Check sheet for the modelled part. Datum: model origin and axes. Units: mm. A direction names the side the tool comes from. Coordinates: 2 decimals unless noted, no trailing zeros. Loops run counter-clockwise (first coordinate to the right, second up) from the corner with the lowest first, then second, coordinate; pieces in that order, holes last.
```python
from build123d import *

# Parameters (mm, degrees)
CROQUIS1_R                               = 7.5
CROQUIS1_R_2                             = 4
SALIENTE_EXTRUIR1_DEPTH                  = 15
CROQUIS2_W                               = 3
CROQUIS2_H                               = 16.302446726
CORTAR_EXTRUIR1_DEPTH                    = 3
SALIENTE_EXTRUIR2_START                  = 5
SALIENTE_EXTRUIR2_DEPTH                  = 5
TALADRO_DE_MARGEN_PARA_M1_61_D           = 1.7
TALADRO_DE_MARGEN_PARA_M1_61_CSINK_D     = 1.75
TALADRO_DE_MARGEN_PARA_M1_61_CSINK_ANGLE = 82
REDONDEO1_R                              = 2
SALIENTE_EXTRUIR3_DEPTH                  = 5


# Read off the part's stored shape, not the designer's step: M14x1.5 Roscas Standard Taladro1
with BuildPart() as part:
    # Croquis1 → Saliente-Extruir1 (new body)
    with BuildSketch(Plane(origin=(0, 0, 0), x_dir=(1, 0, 0), z_dir=(0, 1, 0))):
        with Locations(Location((0, 0, 0), (0, 0, 270))):
            Circle(CROQUIS1_R)
        with Locations(Location((0, 0, 0), (0, 0, 270))):
            Circle(CROQUIS1_R_2, mode=Mode.SUBTRACT)
    extrude(amount=SALIENTE_EXTRUIR1_DEPTH)

    # Croquis2 → Cortar-Extruir1 (cut)
    with BuildSketch(Plane(origin=(0, 15, 0), x_dir=(1, 0, 0), z_dir=(0, 1, 0))):
        Rectangle(CROQUIS2_W, CROQUIS2_H)
    extrude(amount=-CORTAR_EXTRUIR1_DEPTH, mode=Mode.SUBTRACT)

    # M14x1.5 Roscas Standard Taladro1 outline → M14x1.5 Roscas Standard Taladro1 (revolve, cut)
    with BuildSketch(Plane.XY):
        Polygon((6.172, 0), (7.5, 0), (7.5, 10), (7, 10), (7, 0.828), align=None)
    revolve(axis=Axis((0, 0, 0), (0, 1, 0)), mode=Mode.SUBTRACT)

    # Croquis4 → Saliente-Extruir2 (add)
    with BuildSketch(Plane.XZ.offset(SALIENTE_EXTRUIR2_START)):
        with BuildLine():
            ThreePointArc((2.645751311, -3), (3.409321836, -2.092014488), (3.872983346, -1))
            Line((3.872983346, -1), (-3.872983346, -1))
            ThreePointArc((-3.872983346, -1), (-3.409321836, -2.092014488), (-2.645751311, -3))
            Line((-2.645751311, -3), (2.645751311, -3))
        make_face()
        with BuildLine():
            Line((-3.872983346, 1), (3.872983346, 1))
            ThreePointArc((3.872983346, 1), (3.409321836, 2.092014488), (2.645751311, 3))
            Line((2.645751311, 3), (-2.645751311, 3))
            ThreePointArc((-2.645751311, 3), (-3.409321836, 2.092014488), (-3.872983346, 1))
        make_face()
        with BuildLine():
            Line((3.872983346, 1), (5.074404793, 1))
            ThreePointArc((5.074404793, 1), (4.750167411, 2.045847884), (4.213025516, 3))
            Line((4.213025516, 3), (2.645751311, 3))
            ThreePointArc((2.645751311, 3), (3.409321836, 2.092014488), (3.872983346, 1))
        make_face()
        with BuildLine():
            Line((-5.074404793, 1), (-3.872983346, 1))
            ThreePointArc((-3.872983346, 1), (-3.409321836, 2.092014488), (-2.645751311, 3))
            Line((-2.645751311, 3), (-4.213025516, 3))
            ThreePointArc((-4.213025516, 3), (-4.750167411, 2.045847884), (-5.074404793, 1))
        make_face()
        with BuildLine():
            ThreePointArc((4.213025516, -3), (4.750167411, -2.045847884), (5.074404793, -1))
            Line((5.074404793, -1), (3.872983346, -1))
            ThreePointArc((3.872983346, -1), (3.409321836, -2.092014488), (2.645751311, -3))
            Line((2.645751311, -3), (4.213025516, -3))
        make_face()
        with BuildLine():
            ThreePointArc((-2.645751311, -3), (-3.409321836, -2.092014488), (-3.872983346, -1))
            Line((-3.872983346, -1), (-5.074404793, -1))
            ThreePointArc((-5.074404793, -1), (-4.750167411, -2.045847884), (-4.213025516, -3))
            Line((-4.213025516, -3), (-2.645751311, -3))
        make_face()
    extrude(amount=-SALIENTE_EXTRUIR2_DEPTH)

    # Taladro de margen para M1.61 (through all)
    with Locations(Plane(origin=(0, 0, -3), x_dir=(1, 0, 0), z_dir=(0, 0, -1))):
        with Locations((2.65, 2.5), (-2.65, 2.5)):
            CounterSinkHole(TALADRO_DE_MARGEN_PARA_M1_61_D / 2, TALADRO_DE_MARGEN_PARA_M1_61_CSINK_D / 2, counter_sink_angle=TALADRO_DE_MARGEN_PARA_M1_61_CSINK_ANGLE)

    # Redondeo1
    # the kernel refuses this fillet: 2 mm, written as the material it adds along each edge
    with BuildSketch(Plane(origin=(0, 0, 0), x_dir=(0.503234651569935, 0, -0.8641498049871251), z_dir=(0.8641498049871251, 0, 0.503234651569935))) as redondeo1_piece_1_section:
        with BuildLine():
            CenterArc((4 - REDONDEO1_R, REDONDEO1_R), REDONDEO1_R, 270, 90)
            Line((4 - REDONDEO1_R, 0), (4, 0))
            Line((4, 0), (4, REDONDEO1_R))
        make_face()
    redondeo1_piece_1 = revolve(axis=Axis((0, 0, 0), (0, 1, 0)), revolution_arc=177.360579055, mode=Mode.PRIVATE)
    redondeo1_piece_1 = split(redondeo1_piece_1, bisect_by=Plane(origin=(0.549602468, 0.055077536, -1), z_dir=(0, 0, -1)), keep=Keep.TOP, mode=Mode.PRIVATE)
    redondeo1_piece_1 = split(redondeo1_piece_1, bisect_by=Plane(origin=(0.549602468, 0.055077536, -3), z_dir=(0, 0, 1)), keep=Keep.TOP, mode=Mode.PRIVATE)
    add(redondeo1_piece_1)
    with BuildSketch(Plane(origin=(0, 0, 0), x_dir=(0.503234651569935, 0, -0.8641498049871251), z_dir=(0.8641498049871251, 0, 0.503234651569935))) as redondeo1_piece_2_section:
        with BuildLine():
            CenterArc((4 - REDONDEO1_R, REDONDEO1_R), REDONDEO1_R, 270, 90)
            Line((4 - REDONDEO1_R, 0), (4, 0))
            Line((4, 0), (4, REDONDEO1_R))
        make_face()
    redondeo1_piece_2 = revolve(axis=Axis((0, 0, 0), (0, 1, 0)), revolution_arc=177.360579055, mode=Mode.PRIVATE)
    redondeo1_piece_2 = split(redondeo1_piece_2, bisect_by=Plane(origin=(-2.883008057, 0.461894683, 3), z_dir=(0, 0, -1)), keep=Keep.TOP, mode=Mode.PRIVATE)
    redondeo1_piece_2 = split(redondeo1_piece_2, bisect_by=Plane(origin=(-2.883008057, 0.461894683, 1), z_dir=(0, 0, 1)), keep=Keep.TOP, mode=Mode.PRIVATE)
    add(redondeo1_piece_2)
    with BuildSketch(Plane(origin=(0, 0, 0), x_dir=(0.5424951341174628, 0, 0.8400589440383789), z_dir=(-0.8400589440383789, 0, 0.5424951341174628))) as redondeo1_piece_3_section:
        with BuildLine():
            CenterArc((4 - REDONDEO1_R, REDONDEO1_R), REDONDEO1_R, 270, 90)
            Line((4 - REDONDEO1_R, 0), (4, 0))
            Line((4, 0), (4, REDONDEO1_R))
        make_face()
    redondeo1_piece_3 = revolve(axis=Axis((0, 0, 0), (0, 1, 0)), revolution_arc=177.360579055, mode=Mode.PRIVATE)
    redondeo1_piece_3 = split(redondeo1_piece_3, bisect_by=Plane(origin=(2.883008085, 0.461894764, 3), z_dir=(0, 0, -1)), keep=Keep.TOP, mode=Mode.PRIVATE)
    redondeo1_piece_3 = split(redondeo1_piece_3, bisect_by=Plane(origin=(2.883008085, 0.461894764, 1), z_dir=(0, 0, 1)), keep=Keep.TOP, mode=Mode.PRIVATE)
    add(redondeo1_piece_3)
    with BuildSketch(Plane(origin=(0, 0, 0), x_dir=(0.5424951341174628, 0, 0.8400589440383789), z_dir=(-0.8400589440383789, 0, 0.5424951341174628))) as redondeo1_piece_4_section:
        with BuildLine():
            CenterArc((4 - REDONDEO1_R, REDONDEO1_R), REDONDEO1_R, 270, 90)
            Line((4 - REDONDEO1_R, 0), (4, 0))
            Line((4, 0), (4, REDONDEO1_R))
        make_face()
    redondeo1_piece_4 = revolve(axis=Axis((0, 0, 0), (0, 1, 0)), revolution_arc=177.360579055, mode=Mode.PRIVATE)
    redondeo1_piece_4 = split(redondeo1_piece_4, bisect_by=Plane(origin=(3.341819362, 1.478859592, -1), z_dir=(0, 0, -1)), keep=Keep.TOP, mode=Mode.PRIVATE)
    redondeo1_piece_4 = split(redondeo1_piece_4, bisect_by=Plane(origin=(3.341819362, 1.478859592, -3), z_dir=(0, 0, 1)), keep=Keep.TOP, mode=Mode.PRIVATE)
    add(redondeo1_piece_4)
    with BuildSketch(Plane(origin=(0, 0, 0), x_dir=(-0.5032346515699374, 0, 0.8641498049871236), z_dir=(-0.8641498049871236, 0, -0.5032346515699374))) as redondeo1_piece_5_section:
        with BuildLine():
            CenterArc((4 - REDONDEO1_R, REDONDEO1_R), REDONDEO1_R, 270, 90)
            Line((4 - REDONDEO1_R, 0), (4, 0))
            Line((4, 0), (4, REDONDEO1_R))
        make_face()
    redondeo1_piece_5 = revolve(axis=Axis((0, 0, 0), (0, 1, 0)), revolution_arc=177.360579055, mode=Mode.PRIVATE)
    redondeo1_piece_5 = split(redondeo1_piece_5, bisect_by=Plane(origin=(-0.549602468, 0.055077536, 3), z_dir=(0, 0, -1)), keep=Keep.TOP, mode=Mode.PRIVATE)
    redondeo1_piece_5 = split(redondeo1_piece_5, bisect_by=Plane(origin=(-0.549602468, 0.055077536, 1), z_dir=(0, 0, 1)), keep=Keep.TOP, mode=Mode.PRIVATE)
    add(redondeo1_piece_5)
    with BuildSketch(Plane(origin=(0, 0, 0), x_dir=(-0.5032346515699374, 0, 0.8641498049871236), z_dir=(-0.8641498049871236, 0, -0.5032346515699374))) as redondeo1_piece_6_section:
        with BuildLine():
            CenterArc((4 - REDONDEO1_R, REDONDEO1_R), REDONDEO1_R, 270, 90)
            Line((4 - REDONDEO1_R, 0), (4, 0))
            Line((4, 0), (4, REDONDEO1_R))
        make_face()
    redondeo1_piece_6 = revolve(axis=Axis((0, 0, 0), (0, 1, 0)), revolution_arc=177.360579055, mode=Mode.PRIVATE)
    redondeo1_piece_6 = split(redondeo1_piece_6, bisect_by=Plane(origin=(2.883008057, 0.461894683, -1), z_dir=(0, 0, -1)), keep=Keep.TOP, mode=Mode.PRIVATE)
    redondeo1_piece_6 = split(redondeo1_piece_6, bisect_by=Plane(origin=(2.883008057, 0.461894683, -3), z_dir=(0, 0, 1)), keep=Keep.TOP, mode=Mode.PRIVATE)
    add(redondeo1_piece_6)
    with BuildSketch(Plane(origin=(0, 0, 0), x_dir=(-0.542495134117437, 0, -0.8400589440383955), z_dir=(0.8400589440383955, 0, -0.542495134117437))) as redondeo1_piece_7_section:
        with BuildLine():
            CenterArc((4 - REDONDEO1_R, REDONDEO1_R), REDONDEO1_R, 270, 90)
            Line((4 - REDONDEO1_R, 0), (4, 0))
            Line((4, 0), (4, REDONDEO1_R))
        make_face()
    redondeo1_piece_7 = revolve(axis=Axis((0, 0, 0), (0, 1, 0)), revolution_arc=177.360579055, mode=Mode.PRIVATE)
    redondeo1_piece_7 = split(redondeo1_piece_7, bisect_by=Plane(origin=(-2.883008085, 0.461894764, -1), z_dir=(0, 0, -1)), keep=Keep.TOP, mode=Mode.PRIVATE)
    redondeo1_piece_7 = split(redondeo1_piece_7, bisect_by=Plane(origin=(-2.883008085, 0.461894764, -3), z_dir=(0, 0, 1)), keep=Keep.TOP, mode=Mode.PRIVATE)
    add(redondeo1_piece_7)
    with BuildSketch(Plane(origin=(0, 0, 0), x_dir=(-0.542495134117437, 0, -0.8400589440383955), z_dir=(0.8400589440383955, 0, -0.542495134117437))) as redondeo1_piece_8_section:
        with BuildLine():
            CenterArc((4 - REDONDEO1_R, REDONDEO1_R), REDONDEO1_R, 270, 90)
            Line((4 - REDONDEO1_R, 0), (4, 0))
            Line((4, 0), (4, REDONDEO1_R))
        make_face()
    redondeo1_piece_8 = revolve(axis=Axis((0, 0, 0), (0, 1, 0)), revolution_arc=177.360579055, mode=Mode.PRIVATE)
    redondeo1_piece_8 = split(redondeo1_piece_8, bisect_by=Plane(origin=(-3.341819362, 1.478859592, 3), z_dir=(0, 0, -1)), keep=Keep.TOP, mode=Mode.PRIVATE)
    redondeo1_piece_8 = split(redondeo1_piece_8, bisect_by=Plane(origin=(-3.341819362, 1.478859592, 1), z_dir=(0, 0, 1)), keep=Keep.TOP, mode=Mode.PRIVATE)
    add(redondeo1_piece_8)

    # Croquis10 → Saliente-Extruir3 (add)
    with BuildSketch(Plane.XZ):
        with BuildLine():
            ThreePointArc((2.645751311, 3), (0, 4), (-2.645751311, 3))
            Line((-2.645751311, 3), (2.645751311, 3))
        make_face()
        with BuildLine():
            ThreePointArc((-2.645751311, -3), (0, -4), (2.645751311, -3))
            Line((2.645751311, -3), (-2.645751311, -3))
        make_face()
    extrude(amount=-SALIENTE_EXTRUIR3_DEPTH)


solid = part.part
```
1) Section check A-A on y = -1.25. Enter the section's corners in (x, z), plus the area to 3 significant figures.
Answer sheet:
outline: (-5.07, -1) arc R5.17 ccw to (-4.21, -3) - (4.21, -3) arc R5.17 ccw to (5.07, -1) - close; (-5.07, 1) - (5.07, 1) arc R5.17 ccw to (4.21, 3) - (-4.21, 3) arc R5.17 ccw to start
area: 37.8 mm2
2) Set-up check for faces 1 (the flat face through (0, 5, -3.4)), 2 (the flat face through (0, -2, 3)), 3 (the flat face through (0, -2, -3)), 4 (the flat face through (-4.5, 15, -0.1)), 5 (the flat face through (-1.5, 14, -6)): record each of +Z, -Z, +X, -X, +Y, -Y from which the full face is reachable in a straight line by a thin tool's end or side.
Answer sheet:
face 1: +Y
face 2: +Z, +X, -X, -Y
face 3: -Z, +X, -X, -Y
face 4: +Z, -Z, +X, -X, +Y
face 5: +Z, -Z, +Y
3) Section check D-D on y = 9.5. Enter the section's corners in (x, z), plus the area to 3 significant figures.
Answer sheet:
outline: circle Ø14 at (0, 0); hole circle Ø8 at (0, 0)
area: 104 mm2
4) Depth check by flat-ended pin: pin 1 (1.5 mm diameter, centred on y = 9.5, z = -5, fed in from -X); pin 2 (0.8 mm diameter, centred on x = -0.5, z = -1.5, fed in from +Y); pin 3 (0.8 mm diameter, centred on x = 0.5, z = -3.5, fed in from +Y); pin 4 (1.4 mm diameter, centred on x = 2.65, y = -2.5, fed in from +Z). Enter the tip coordinate at first touch or a pass-through.
Answer sheet:
pin 1: stops at x = -6.04
pin 2: stops at y = 0
pin 3: stops at y = 5
pin 4: passes through
5) Section check B-B on y = 4. Enter the section's corners in (x, z).
Answer sheet:
outline: circle Ø14 at (0, 0); hole (-2.65, -3) - (2.65, -3) arc R4 ccw to (2.65, 3) - (-2.65, 3) arc R4 ccw to start
6) Section check C-C on z = -1.25. Give the number of separate pieces and of enclosed holes in the cut face, plus the area to 3 significant figures.
Answer sheet:
separate pieces: 1
enclosed holes: 2
area: 145 mm2
7) Mould release check, pull along X, two halves, no side actions. Record for faces 6 (the flat face through (-1.5, 14, 6)), 7 (the flat face through (0, -5, 2)), 8 (the cylindrical face through (-4.756, -2.535, -2.032)): +X half, -X half, draft (parallel to the pull), parting line (faces both ways), or undercut.
Answer sheet:
face 6: undercut
face 7: draft
face 8: -X half
8) Scan lines: line 1 (Y direction, x = 2.65, z = -2.4); line 2 (X direction, y = -2.5, z = -2.3); line 3 (Z direction, x = 0, y = 5.5). Record each from-to range of solid material in increasing order.
Answer sheet:
line 1: y = -5 to -3.35, -1.65 to 0.77
line 2: x = -4.63 to -3.5, -1.8 to 1.8, 3.5 to 4.63
line 3: z = -7 to -4, 4 to 7
